```python
from build123d import *

# Parameters (mm, degrees)
BOSS_EXTRU_1_DEPTH      = 12.7
ENL_V_MAT_EXTRU_1_DEPTH = 13.7


with BuildPart() as part:
    # Esquisse1 → Boss.-Extru.1 (new body)
    with BuildSketch(Plane(origin=(0, 0, 0), x_dir=(1, 0, 0), z_dir=(0, 1, 0))):
        with BuildLine():
            Line((-357.5, 367.5), (357.5, 367.5))
            ThreePointArc((357.5, 367.5), (364.571067812, 364.571067812), (367.5, 357.5))
            Line((367.5, 357.5), (367.5, -357.5))
            ThreePointArc((367.5, -357.5), (364.571067812, -364.571067812), (357.5, -367.5))
            Line((357.5, -367.5), (-357.5, -367.5))
            ThreePointArc((-357.5, -367.5), (-364.571067812, -364.571067812), (-367.5, -357.5))
            Line((-367.5, -357.5), (-367.5, 357.5))
            ThreePointArc((-367.5, 357.5), (-364.571067812, 364.571067812), (-357.5, 367.5))
        make_face()
    extrude(amount=BOSS_EXTRU_1_DEPTH)

    # Esquisse2 → Enlèv. mat.-Extru.1 (cut, through all)
    with BuildSketch(Plane(origin=(0, 12.7, 0), x_dir=(1, 0, 0), z_dir=(0, 1, 0))):
        with BuildLine():
            ThreePointArc((26, 0), (0, 26), (-26, 0))
            ThreePointArc((-26, 0), (-30, -4), (-34, 0))
            ThreePointArc((-34, 0), (0, 34), (34, 0))
            ThreePointArc((34, 0), (-30, -64), (-94, 0))
            ThreePointArc((-94, 0), (0, 94), (94, 0))
            ThreePointArc((94, 0), (-30, -124), (-154, 0))
            ThreePointArc((-154, 0), (0, 154), (154, 0))
            ThreePointArc((154, 0), (-30, -184), (-214, 0))
            ThreePointArc((-214, 0), (0, 214), (214, 0))
            ThreePointArc((214, 0), (-30, -244), (-274, 0))
            ThreePointArc((-274, 0), (0, 274), (274, 0))
            ThreePointArc((274, 0), (-30, -304), (-334, 0))
            ThreePointArc((-334, 0), (0, 334), (334, 0))
            ThreePointArc((334, 0), (330, -4), (326, 0))
            ThreePointArc((326, 0), (0, 326), (-326, 0))
            ThreePointArc((-326, 0), (-30, -296), (266, 0))
            ThreePointArc((266, 0), (0, 266), (-266, 0))
            ThreePointArc((-266, 0), (-30, -236), (206, 0))
            ThreePointArc((206, 0), (0, 206), (-206, 0))
            ThreePointArc((-206, 0), (-30, -176), (146, 0))
            ThreePointArc((146, 0), (0, 146), (-146, 0))
            ThreePointArc((-146, 0), (-30, -116), (86, 0))
            ThreePointArc((86, 0), (0, 86), (-86, 0))
            ThreePointArc((-86, 0), (-30, -56), (26, 0))
        make_face()
    extrude(amount=-ENL_V_MAT_EXTRU_1_DEPTH, mode=Mode.SUBTRACT)


solid = part.part
```
Work out the finished part from the listing and answer in its coordinate system (mm). Coordinates: 2 decimals unless noted, no trailing zeros. Order: outer loops, then holes, each group sorted by start corner. A loop starts at its lowest first (then second) coordinate and runs counter-clockwise, first axis right, second up. Notation, with made-up numbers: M 27,6.25 L 64,6.25 A22 ccw 64,27.25 Z; hole C 3,23.25 d9. An arc over 180 degrees is marked long. Use CSV: the item, a comma, the result in double quotes.
1) Section D-D on x = 0 is taken. Count the separate pieces of the cut face and the enclosed holes in it, plus the area to 3 significant figures.
Worked out:
separate pieces,"12"
enclosed holes,"0"
area,"8,190 mm^2"
2) Section B-B on x = 312 is taken. Write down the section's boundary in (y, z).
Worked out:
outline,"M 0,-367.5 L 12.7,-367.5 L 12.7,-119.21 L 0,-119.21 Z; M 0,-94.51 L 12.7,-94.51 L 12.7,367.5 L 0,367.5 Z"
3) Determine the mould class of faces 1 (the face through (5, 12.7, -5)), 2 (the face through (-23.315, 6.439, 303.926)) for opening direction Z: released by +Z, released by -Z, zero draft, split by the parting line, or undercut.
Worked out:
face 1,"zero draft"
face 2,"undercut"
4) Consider line 1 (X direction, y = 7, z = -226.5); line 2 (Z direction, x = 187, y = 11). Determine where each line is inside the solid, lowest interval first. Write a range as [from, to].
Worked out:
line 1,"x = [-367.5, -245.47], [-234.46, -154.19], [-139.48, 139.48], [154.19, 234.46], [245.47, 367.5]"
line 2,"z = [-367.5, -276.74], [-267.03, -200.27], [-189.17, -104.05], [-86.41, 92.77], [111.57, 201.31], [212.9, 367.5]"
5) Section C-C on x = -231 is taken. Write down the section's boundary in (y, z), plus the area to 3 significant figures.
Worked out:
outline,"M 0,-367.5 L 12.7,-367.5 L 12.7,-241.24 L 0,-241.24 Z; M 0,-230.03 L 12.7,-230.03 L 12.7,-147.36 L 0,-147.36 Z; M 0,-131.89 L 12.7,-131.89 L 12.7,123.67 L 0,123.67 Z; M 0,138.33 L 12.7,138.33 L 12.7,217.29 L 0,217.29 Z; M 0,228.07 L 12.7,228.07 L 12.7,367.5 L 0,367.5 Z"
area,"8,670 mm^2"
